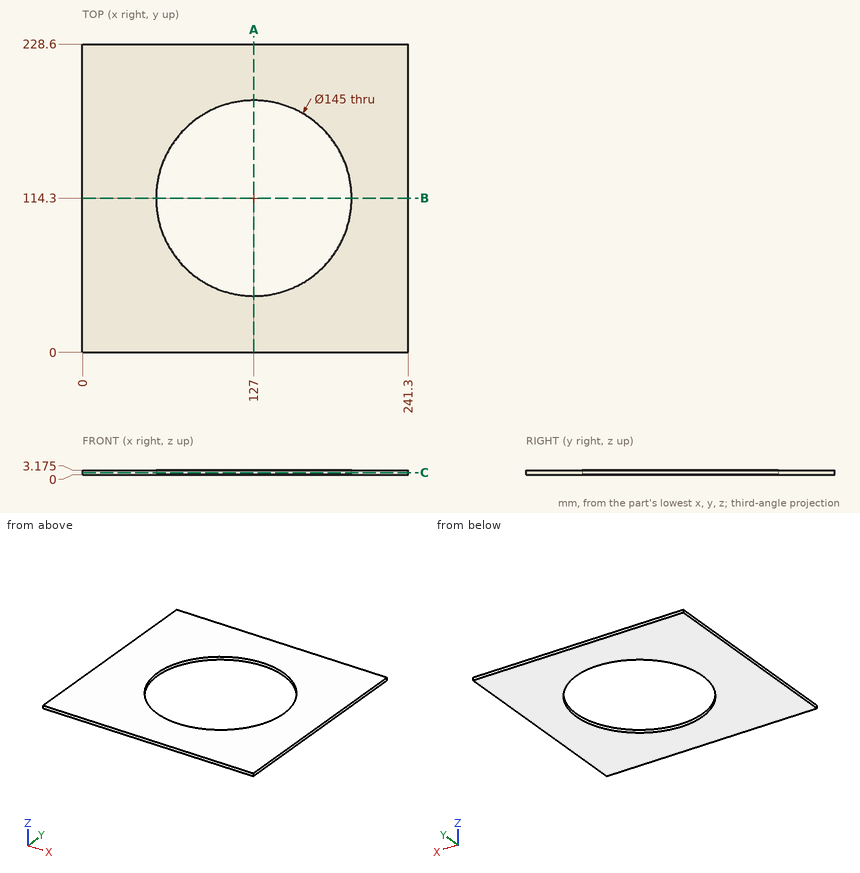
Answer from the drawing. Dimensions are ordinates in mm from the lowest x, y and z of the part. Give positions to 0.01 mm unless a question says otherwise; leave off trailing zeros. Loops run counter-clockwise (first coordinate to the right, second up) from the corner with the lowest first, then second, coordinate; pieces in that order, holes last. Notation, with made-up numbers: (51, 82.5) - (109, 82.5) arc R21 ccw to (109, 101.5) - close; hole circle Ø1 at (-1.5, -38). An arc over 180 degrees is marked (long way). Answer as CSV lines item,"result". Start each with the question number.
Item 1: A cutting plane is placed at A-A on x = 127. Determine the outline of the cut face in (y, z) (3 decimals).
Item 2: A cutting plane is placed at B-B on y = 114.3. Determine the outline of the cut face in (x, z) (3 decimals).
Item 3: A cutting plane is placed at C-C on z = 1.5. Determine the outline of the cut face in (x, y).
Item 4: Find the intervals of material crossed by line 1 (Y direction, x = 127, z = 1.4); line 2 (X direction, y = 131.5, z = 1.45); line 3 (X direction, y = 142, z = 0.35), in increasing order. Write a range as from..to.
Found:
1,outline,"(0, 0) - (41.8, 0) - (41.8, 3.175) - (0, 3.175) - close; (186.8, 0) - (228.6, 0) - (228.6, 3.175) - (186.8, 3.175) - close"
2,outline,"(0, 0) - (54.5, 0) - (54.5, 3.175) - (0, 3.175) - close; (199.5, 0) - (241.3, 0) - (241.3, 3.175) - (199.5, 3.175) - close"
3,outline,"(0, 0) - (241.3, 0) - (241.3, 228.6) - (0, 228.6) - close; hole circle Ø145 at (127, 114.3)"
4,line 1,"y = 0..41.8, 186.8..228.6"
4,line 2,"x = 0..56.57, 197.43..241.3"
4,line 3,"x = 0..60, 194..241.3"
